Can you work these out from the model? Positions are in its coordinate system, mm. A direction names the side the tool comes from. Round coordinates to 2 decimals unless told otherwise and drop trailing zeros. Write each loop counter-clockwise with the first axis right and the second up, starting at its lowest first coordinate (ties: lowest second). Pieces come first, ordered by that corner, then holes. Notation, with made-up numbers: M 4,42.25 L 16,42.25 A6 ccw 16,52.25 Z; hole C -37,-8 d2. An arc over 180 degrees is marked long. Answer as a JSON object with one key per item and string values. Group by question number.
1) Please list where these lines run through material, in increasing order: L1, parallel to Z at x = 30.5, y = -25; L2, parallel to Y at x = 5, z = 37; L3, parallel to Z at x = 2.8, y = 0. Write a range as [from, to].
2) Suppose I cut it at B-B, the plane x = 15. Write out the boundary of the cut face in (y, z).
3) Suppose I cut it at D-D, the plane y = 23. Write out the boundary of the cut face in (x, z) (3 decimals).
4) If we mould it in two halves opening along Y, with no side actions, what happens to faces 4 (the flat face through (3, 32, 5)), 5 (the cylindrical face through (2.788, 34.023, -42.076)), 6 (the flat face through (5.5, 0, -54))? For each: +Y half, -Y half, draft (parallel to the pull), parting line (faces both ways), or undercut.
5) Suppose I cut it at C-C, the plane y = 0. Write out the boundary of the cut face in (x, z) (3 decimals).
6) Suppose I cut it at A-A, the plane z = 0. Write out the boundary of the cut face in (x, y), and give its area (3 significant figures).
7) On a 3-axis mill with a long thin cutter (end or side, diameter ignored), from which of +Z, -Z, +X, -X, +Y, -Y can I reach the whole of each face in a straight line? I mean faces 1 (the flat face through (3, 32, -5)), 2 (the flat face through (42.477, -0.619, 42.84)), 3 (the cylindrical face through (2.788, -34.023, -33.674)). Say none if no direction works.
8) I'm going to push flat-ended pins straight in: pin 1 Ø5.5 at (y, z) = (0, 55) entering from +X; pin 2 Ø8 at (x, y) = (24, -19) entering from -Z; pin 3 Ø1.6 at (x, y) = (44.5, -17) entering from +Z. Where does each tip first touch, or does it pass through?
from build123d import *

# Parameters (mm, degrees)
SKETCH1_R           = 60.5
BOSS_EXTRUDE1_DEPTH = 5.5
SKETCH2_R           = 5.7
SKETCH2_R_2         = 25
CUT_EXTRUDE1_DEPTH  = 86.736514975
BOSS_EXTRUDE2_DEPTH = 38.1
BOSS_EXTRUDE3_DEPTH = 5
CHAMFER1_SIZE       = 10
CHAMFER1_SIZE_2     = 3.639702343
CHAMFER2_SIZE       = 10
CHAMFER2_SIZE2      = 3.639702343
CHAMFER3_SIZE       = 1.819851171
CHAMFER3_SIZE_2     = 5
CHAMFER4_SIZE       = 5
CHAMFER4_SIZE_2     = 1.819851171
FILLET1_R           = 5
CHAMFER5_SIZE       = 3.213333015
CHAMFER5_SIZE_2     = 2.25
CHAMFER6_SIZE       = 2.25
CHAMFER6_SIZE_2     = 3.213333015
SKETCH5_R           = 6
CUT_EXTRUDE2_DEPTH  = 96.112299108


with BuildPart() as part:
    # Sketch1 → Boss-Extrude1 (new body)
    with BuildSketch(Plane(origin=(0, 0, 0), x_dir=(0, 0, -1), z_dir=(1, 0, 0))):
        Circle(SKETCH1_R)
    extrude(amount=BOSS_EXTRUDE1_DEPTH)

    # Sketch2 → Cut-Extrude1 (cut, through all)
    with BuildSketch(Plane(origin=(5.5, 0, 0), x_dir=(0, 0, -1), z_dir=(1, 0, 0))):
        with Locations((-37.875, 37.875)):
            Circle(SKETCH2_R)
        with Locations(Location((37.875, 37.875, 0), (0, 0, 180))):
            Circle(SKETCH2_R)
        with Locations((37.875, -37.875)):
            Circle(SKETCH2_R)
        with Locations(Location((-37.875, -37.875, 0), (0, 0, 180))):
            Circle(SKETCH2_R)
        Circle(SKETCH2_R_2)
    extrude(amount=-CUT_EXTRUDE1_DEPTH, mode=Mode.SUBTRACT)

    # Sketch3 → Boss-Extrude2 (add)
    with BuildSketch(Plane(origin=(5.5, 0, 0), x_dir=(0, 0, -1), z_dir=(1, 0, 0))):
        with BuildLine():
            ThreePointArc((-44.45, 41.042021149), (-47.05176845, 38.03131717), (-49.45, 34.856097028))
            Line((-49.45, 34.856097028), (-49.45, -34.856097028))
            ThreePointArc((-49.45, -34.856097028), (-47.05176845, -38.03131717), (-44.45, -41.042021149))
            Line((-44.45, -41.042021149), (-44.45, 41.042021149))
        make_face()
        with BuildLine():
            ThreePointArc((49.45, 34.856097028), (47.05176845, 38.03131717), (44.45, 41.042021149))
            Line((44.45, 41.042021149), (44.45, -41.042021149))
            ThreePointArc((44.45, -41.042021149), (47.05176845, -38.03131717), (49.45, -34.856097028))
            Line((49.45, -34.856097028), (49.45, 34.856097028))
        make_face()
    extrude(amount=BOSS_EXTRUDE2_DEPTH)

    # Sketch4 → Boss-Extrude3 (add)
    with BuildSketch(Plane(origin=(43.6, 0, 0), x_dir=(0, 0, -1), z_dir=(1, 0, 0))):
        with BuildLine():
            Line((-41.275, -44.233747015), (-41.275, 44.233747015))
            ThreePointArc((-41.275, 44.233747015), (-42.892198414, 42.667426865), (-44.45, 41.042021149))
            Line((-44.45, 41.042021149), (-44.45, -41.042021149))
            ThreePointArc((-44.45, -41.042021149), (-42.892198414, -42.667426865), (-41.275, -44.233747015))
        make_face()
        with BuildLine():
            Line((-49.45, 34.856097028), (-49.45, -34.856097028))
            ThreePointArc((-49.45, -34.856097028), (-47.05176845, -38.03131717), (-44.45, -41.042021149))
            Line((-44.45, -41.042021149), (-44.45, 41.042021149))
            ThreePointArc((-44.45, 41.042021149), (-47.05176845, 38.03131717), (-49.45, 34.856097028))
        make_face()
        with BuildLine():
            Line((49.45, -34.856097028), (49.45, 34.856097028))
            ThreePointArc((49.45, 34.856097028), (45.604182769, 39.755609842), (41.275, 44.233747015))
            Line((41.275, 44.233747015), (41.275, -44.233747015))
            ThreePointArc((41.275, -44.233747015), (45.604182769, -39.755609842), (49.45, -34.856097028))
        make_face()
    extrude(amount=BOSS_EXTRUDE3_DEPTH)

    # Chamfer1
    # the kernel refuses this chamfer: 10, 3.639702343 mm, written as the material it takes off along each edge
    with BuildSketch(Plane(origin=(48.6, 60.798044353, 49.45), x_dir=(-0.9999130865277315, 0, 0.013184058198646176), z_dir=(0, -1, 0))) as chamfer1_piece_1:
        Polygon((CHAMFER1_SIZE * 0.999913086528, CHAMFER1_SIZE * 0.0131840581986), (-CHAMFER1_SIZE_2 * 0.0131840581974, CHAMFER1_SIZE_2 * 0.999913086435), (0, 0), align=None)
    extrude(amount=121.596088706, mode=Mode.SUBTRACT)

    # Chamfer2
    chamfer2_edges = [part.edges().sort_by_distance(p)[0] for p in [
        (48.6, 0, -49.45),
    ]]
    chamfer2_side = [part.faces().sort_by_distance(p)[0] for p in [
        (27.05, 0, -49.45),
    ]]
    chamfer(chamfer2_edges, length=CHAMFER2_SIZE, length2=CHAMFER2_SIZE2, reference=chamfer2_side[0])

    # Chamfer3
    # the kernel refuses this chamfer: 5, 1.819851171 mm, written as the material it takes off along each edge
    with BuildSketch(Plane(origin=(48.6, -57.204720678, 41.275), x_dir=(-0.9950833631817487, 0, -0.09904090225204971), z_dir=(0, 1, 0))) as chamfer3_piece_1:
        Polygon((CHAMFER3_SIZE * 0.995083363363, CHAMFER3_SIZE * 0.0990409022701), (-CHAMFER3_SIZE_2 * 0.099040902252, CHAMFER3_SIZE_2 * 0.995083363182), (0, 0), align=None)
    extrude(amount=114.409441356, mode=Mode.SUBTRACT)

    # Chamfer4
    # the kernel refuses this chamfer: 5, 1.819851171 mm, written as the material it takes off along each edge
    with BuildSketch(Plane(origin=(48.6, 57.204720678, -41.275), x_dir=(0.013184058198646176, 0, -0.9999130865277315), z_dir=(0, -1, 0))) as chamfer4_piece_1:
        Polygon((CHAMFER4_SIZE * 0.999913086528, -CHAMFER4_SIZE * 0.0131840581986), (-CHAMFER4_SIZE_2 * 0.013184058201, -CHAMFER4_SIZE_2 * 0.99991308671), (0, 0), align=None)
    extrude(amount=114.409441356, mode=Mode.SUBTRACT)

    # Fillet1
    # the kernel refuses this fillet: 5 mm, written as the material it takes off along each edge
    with BuildSketch(Plane(origin=(48.450647546, -51.951472504, -45.864657505), x_dir=(-0.9396926207859081, 0, -0.34202014332566955), z_dir=(0, 1, 0))) as fillet1_piece_1:
        with BuildLine():
            CenterArc((4.998659123, 5), FILLET1_R, 181.326957093, 88.673042907)
            Line((0, 4.8842115), (-0.099973182, 4.88189573))
            ThreePointArc((-0.099973182, 4.88189573), (-0.1, 2.44210575), (-0.1, 0))
            Line((-0.1, 0), (0, -0.1))
            Line((0, -0.1), (4.998659123, -0.1))
            Line((4.998659123, -0.1), (4.998659123, 0))
        make_face()
    extrude(amount=103.902945009, mode=Mode.SUBTRACT)
    with BuildSketch(Plane(origin=(48.450647546, -51.951472504, 45.864657505), x_dir=(-0.9396926207857893, 0, 0.3420201433259962), z_dir=(0, 1, 0))) as fillet1_piece_2:
        with BuildLine():
            CenterArc((4.998659123, -5), FILLET1_R, 90, 88.673042907)
            Line((0, -4.8842115), (-0.099973182, -4.88189573))
            ThreePointArc((-0.099973182, -4.88189573), (-0.1, -2.44210575), (-0.1, 0))
            Line((-0.1, 0), (0, 0.1))
            Line((0, 0.1), (4.998659123, 0.1))
            Line((4.998659123, 0.1), (4.998659123, 0))
        make_face()
    extrude(amount=103.902945009, mode=Mode.SUBTRACT)

    # Chamfer5
    # the kernel refuses this chamfer: 3.213333015, 2.25 mm, written as the material it adds along each edge
    with BuildSketch(Plane(origin=(43.6, -49.340621494, 44.45), x_dir=(0.02220967419845722, 0, -0.99975333476413), z_dir=(0, 1, 0))) as chamfer5_piece_1_section:
        Polygon((CHAMFER5_SIZE * 0.999753334817, CHAMFER5_SIZE * 0.0222096741996), (-CHAMFER5_SIZE_2 * 0.0222096741985, CHAMFER5_SIZE_2 * 0.999753334764), (0, 0), align=None)
    chamfer5_piece_1 = extrude(amount=98.681242988, mode=Mode.PRIVATE)
    chamfer5_piece_1 = chamfer5_piece_1 & Plane(origin=(42.872647852, 0, 0), x_dir=(0, 0, -1), z_dir=(-1, 0, 0)) * Cylinder(60.5, 211, mode=Mode.PRIVATE)
    chamfer5_piece_1 = split(chamfer5_piece_1, bisect_by=Plane(origin=(42.872647852, 1e-09, 41.275), z_dir=(0, 0, 1)), keep=Keep.TOP, mode=Mode.PRIVATE)
    add(chamfer5_piece_1)

    # Chamfer6
    # the kernel refuses this chamfer: 3.213333015, 2.25 mm, written as the material it adds along each edge
    with BuildSketch(Plane(origin=(43.6, 49.340621494, -44.45), x_dir=(-0.9989750717851553, 0, -0.04526373771402063), z_dir=(0, -1, 0))) as chamfer6_piece_1_section:
        Polygon((CHAMFER6_SIZE * 0.998975071785, -CHAMFER6_SIZE * 0.045263737714), (-CHAMFER6_SIZE_2 * 0.0452637377164, -CHAMFER6_SIZE_2 * 0.998975071838), (0, 0), align=None)
    chamfer6_piece_1 = extrude(amount=98.681242988, mode=Mode.PRIVATE)
    chamfer6_piece_1 = chamfer6_piece_1 & Plane(origin=(42.872647852, 0, 0), x_dir=(0, 0, -1), z_dir=(-1, 0, 0)) * Cylinder(60.5, 211, mode=Mode.PRIVATE)
    chamfer6_piece_1 = split(chamfer6_piece_1, bisect_by=Plane(origin=(42.872647852, -1e-09, -41.275), z_dir=(0, 0, -1)), keep=Keep.TOP, mode=Mode.PRIVATE)
    add(chamfer6_piece_1)

    # Sketch5 → Cut-Extrude2 (cut, through all)
    with BuildSketch(Plane(origin=(5.5, 0, 0), x_dir=(0, 0, -1), z_dir=(1, 0, 0))):
        with Locations((0, 57.537769206)):
            Circle(SKETCH5_R)
        Polygon((0, 0), (-6.25, 40), (6.25, 40), align=None)
    extrude(amount=-CUT_EXTRUDE2_DEPTH, mode=Mode.SUBTRACT)


solid = part.part
Results:
{
 "1": {"L1": "[-49.45, -44.45], [44.45, 49.45]", "L2": "[-47.87, -43.51], [-32.24, 32.24], [43.51, 47.87]", "L3": "[-60.5, -25], [25, 60.5]"},
 "2": {"outline": "M -41.04,-44.45 A60.5 ccw -34.86,-49.45 L 34.86,-49.45 A60.5 ccw 41.04,-44.45 Z; M -41.04,44.45 L 41.04,44.45 A60.5 ccw 34.86,49.45 L -34.86,49.45 A60.5 ccw Z"},
 "3": {"outline": "M 0,-55.958 L 5.5,-55.958 L 5.5,-49.45 L 38.6,-49.45 L 43.753,-47.574 A5 ccw 46.78,-41.275 L 43.573,-41.275 L 41.35,-44.45 L 5.5,-44.45 L 5.5,-9.798 L 0,-9.798 Z; M 0,9.798 L 5.5,9.798 L 5.5,44.45 L 41.35,44.45 L 43.573,41.275 L 46.78,41.275 A5 ccw 43.753,47.574 L 38.6,49.45 L 5.5,49.45 L 5.5,55.958 L 0,55.958 Z"},
 "4": {"face 4": "undercut", "face 5": "undercut", "face 6": "draft"},
 "5": {"outline": "M 0,-60.5 L 5.5,-60.5 L 5.5,-49.45 L 38.6,-49.45 L 43.753,-47.574 A5 ccw 46.78,-41.275 L 43.573,-41.275 L 41.35,-44.45 L 5.5,-44.45 L 5.5,-25 L 0,-25 Z; M 0,25 L 5.5,25 L 5.5,44.45 L 41.35,44.45 L 43.573,41.275 L 46.78,41.275 A5 ccw 43.753,47.574 L 38.6,49.45 L 5.5,49.45 L 5.5,60.5 L 0,60.5 Z"},
 "6": {"outline": "M 0,-60.5 L 5.5,-60.5 L 5.5,-25 L 0,-25 Z; M 0,40 L 5.5,40 L 5.5,51.54 L 0,51.54 Z", "area": "259 mm^2"},
 "7": {"face 1": "+X, -X", "face 2": "+Y, -Y", "face 3": "-X"},
 "8": {"pin 1": "x = 5.5", "pin 2": "z = -49.45", "pin 3": "z = 47.59"}
}
